Can you work these out from the model? Positions are in its coordinate system, mm. A direction names the side the tool comes from. Give positions to 0.01 mm unless a question says otherwise; leave off trailing zeros. Order: outer loops, then holes, each group sorted by start corner. A loop starts at its lowest first (then second) coordinate and runs counter-clockwise, first axis right, second up. Notation, with made-up numbers: M 87.25,-27 L 116.25,-27 A20 ccw 116.25,-23 Z; hole C -26.75,-28 d4. An arc over 180 degrees is marked long. One line per question, with ' | ' between items. Start each with the question number.
1) If we section it at D-D, the plane z = 98: Please give me the cut outline in (x, y) (3 decimals), plus the area to 3 significant figures.
2) For faces 4 (the cylindrical face through (0.228, 1.479, 8.265)), 5 (the cylindrical face through (0, 5, 47)), which set-ups out of +Z, -Z, +X, -X, +Y, -Y let a thin tool reach every point of the face, with its end or its side?
3) If we section it at C-C, the plane x = 0: State how many separate pieces and enclosed holes the cut face has, plus the area to 4 significant figures.
4) If we section it at A-A, the plane z = 50: Please give me the cut outline in (x, y) (3 decimals).
5) If we section it at B-B, the plane y = 1.25: Please give me the cut outline in (x, z).
6) I'm going to push flat-ended pins straight in: pin 1 Ø5 at (x, z) = (0, 130) entering from +Y; pin 2 Ø2 at (x, z) = (0, 10) entering from +Y. Where does each tip first touch, or does it pass through?
7) Please list where these lines run through material, in increasing order: line 1 along Y through (x, z) = (-3.5, 15) (3 decimals); line 2 along X through (y, z) = (1.2, 50); line 3 along X through (y, z) = (5.25, 10). Write a range as [from, to].
8) Thinking about a two-plate mould opening in Z: for faces 1 (the flat face through (-4.5, 2, 69)), 2 (the flat face through (0, 3, 0)), 3 (the cylindrical face through (-0.65, 4.77, 92.93)), which applies, +Z half, -Z half, draft (parallel to the pull), parting line (faces both ways), or undercut?
```python
from build123d import *

# Parameters (mm, degrees)
EXTRUDE_1_DEPTH           = 140
HOLE_WIZARD_1_D           = 3.5
HOLE_WIZARD_1_CBORE_D     = 6
HOLE_WIZARD_1_CBORE_DEPTH = 3.5
PATTERN_LINEAR_1_COUNT    = 7
PATTERN_LINEAR_1_PITCH    = 20


with BuildPart() as part:
    # 草图1 → 凸台-拉伸1 (new body)
    with BuildSketch(Plane.XY):
        Polygon((4.3, 0), (4.5, 0.2), (4.5, 3), (3.875, 3.625), (3.125, 3.625), (3.125, 4.375), (3.875, 4.375), (4.5, 5), (4.5, 6.3), (4.3, 6.5), (-4.3, 6.5), (-4.5, 6.3), (-4.5, 5), (-3.875, 4.375), (-3.125, 4.375), (-3.125, 3.625), (-3.875, 3.625), (-4.5, 3), (-4.5, 0.2), (-4.3, 0), align=None)
    extrude(amount=EXTRUDE_1_DEPTH)

    # 打孔尺寸(%根据)内六角圆柱头螺钉的类型1 (through all)
    with Locations(Plane(origin=(0, 6.5, 0), x_dir=(1, 0, 0), z_dir=(0, 1, 0))):
        with Locations((0, -10)):
            hole_wizard_1 = CounterBoreHole(HOLE_WIZARD_1_D / 2, HOLE_WIZARD_1_CBORE_D / 2, HOLE_WIZARD_1_CBORE_DEPTH)

    # 阵列(线性)1: 打孔尺寸(%根据)内六角圆柱头螺钉的类型1 ×7
    with Locations(*[(0, 0, i * PATTERN_LINEAR_1_PITCH) for i in range(1, PATTERN_LINEAR_1_COUNT)]):
        add(hole_wizard_1, mode=Mode.SUBTRACT)


solid = part.part
```
Results found:
1) outline: M -4.5,0.2 L -4.3,0 L 4.3,0 L 4.5,0.2 L 4.5,3 L 3.875,3.625 L 3.125,3.625 L 3.125,4.375 L 3.875,4.375 L 4.5,5 L 4.5,6.3 L 4.3,6.5 L -4.3,6.5 L -4.5,6.3 L -4.5,5 L -3.875,4.375 L -3.125,4.375 L -3.125,3.625 L -3.875,3.625 L -4.5,3 Z | area: 55.6 mm²
2) face 4: +Y, -Y | face 5: +Y
3) separate pieces: 8 | enclosed holes: 0 | area: 689.5 mm²
4) outline: M -4.5,0.2 L -4.3,0 L -1.75,0 L -1.75,3 L -3,3 L -3,6.5 L -4.3,6.5 L -4.5,6.3 L -4.5,5 L -3.875,4.375 L -3.125,4.375 L -3.125,3.625 L -3.875,3.625 L -4.5,3 Z; M 1.75,0 L 4.3,0 L 4.5,0.2 L 4.5,3 L 3.875,3.625 L 3.125,3.625 L 3.125,4.375 L 3.875,4.375 L 4.5,5 L 4.5,6.3 L 4.3,6.5 L 3,6.5 L 3,3 L 1.75,3 Z
5) outline: M -4.5,0 L 4.5,0 L 4.5,140 L -4.5,140 Z; hole C 0,10 d3.5; hole C 0,30 d3.5; hole C 0,50 d3.5; hole C 0,70 d3.5; hole C 0,90 d3.5; hole C 0,110 d3.5; hole C 0,130 d3.5
6) pin 1: stops at y = 3 | pin 2: passes through
7) line 1: y = [0, 3.625], [4.375, 6.5] | line 2: x = [-4.5, -1.75], [1.75, 4.5] | line 3: x = [-4.5, -3], [3, 4.5]
8) face 1: draft | face 2: -Z half | face 3: undercut
